Drawing for the job (mm, zero at the part's lowest x, y, z). Round coordinates to 2 decimals unless told otherwise and drop trailing zeros. Loops run counter-clockwise (first coordinate to the right, second up) from the corner with the lowest first, then second, coordinate; pieces in that order, holes last. Notation, with made-up numbers: (24.5, -37.5) - (37.5, -37.5) arc R10 cw to (37.5, -20.5) - close; hole circle Ø6 at (24, 29). An arc over 180 degrees is marked (long way). Put each result on its own line as item: value.
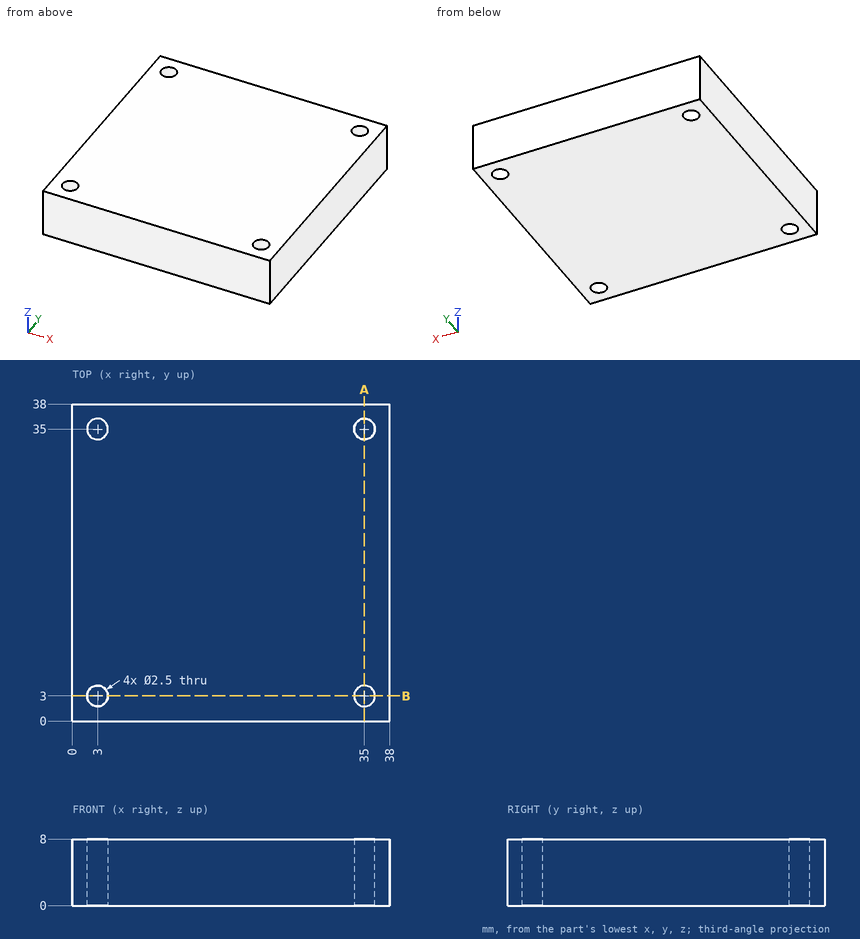
1. Probe line 1 along X through (y, z) = (3, 6.75); line 2 along Y through (x, z) = (34, 1.5). List the from-to ranges inside material, lowest first. Write a range as [from, to].
A:
line 1: x = [0, 1.75], [4.25, 33.75], [36.25, 38]
line 2: y = [0, 2.25], [3.75, 34.25], [35.75, 38]
2. Pin check, flat tip, straight feed: P1, Ø2, axis at x = 3, y = 3, coming from the -Z side. Stop position of the tip, or through.
A:
P1: passes through
3. Band-saw the part on A-A (x = 35). List the corners of the cut face in (y, z), plus the area to 3 significant figures.
A:
outline: (0, 0) - (1.75, 0) - (1.75, 8) - (0, 8) - close; (4.25, 0) - (33.75, 0) - (33.75, 8) - (4.25, 8) - close; (36.25, 0) - (38, 0) - (38, 8) - (36.25, 8) - close
area: 264 mm²
